Answer from the drawing. Dimensions are ordinates in mm from the lowest x, y and z of the part. Coordinates: 2 decimals unless noted, no trailing zeros. Write each loop counter-clockwise with the first axis right and the second up, starting at its lowest first coordinate (ties: lowest second). Pieces come first, ordered by that corner, then holes.
(1) Section A-A on y = 97.5 is taken. Write down the section's boundary in (x, z), then the cut area to 3 significant figures.
(2) Given pin 1 (3 mm diameter, centred on y = 81.5, z = 403, fed in from +X); pin 2 (4 mm diameter, centred on x = 120.5, z = 214, fed in from +Y), each flat-ended and moving along its own axis, determine where each tip first touches the part or whether it passes through.
(3) Section C-C on z = 207 is taken. Write down the section's boundary in (x, y), then the cut area to 3 significant figures.
(4) Find the intervals of material crossed by probe 1 along Y at (x, z) = (65, 88); probe 2 along Z at (x, y) = (142, 45.5); probe 3 along Z at (x, y) = (118, 10), in increasing order.
(5) Section B-B on x = 33 is taken. Write down the section's boundary in (y, z), then the cut area to 3 significant figures.
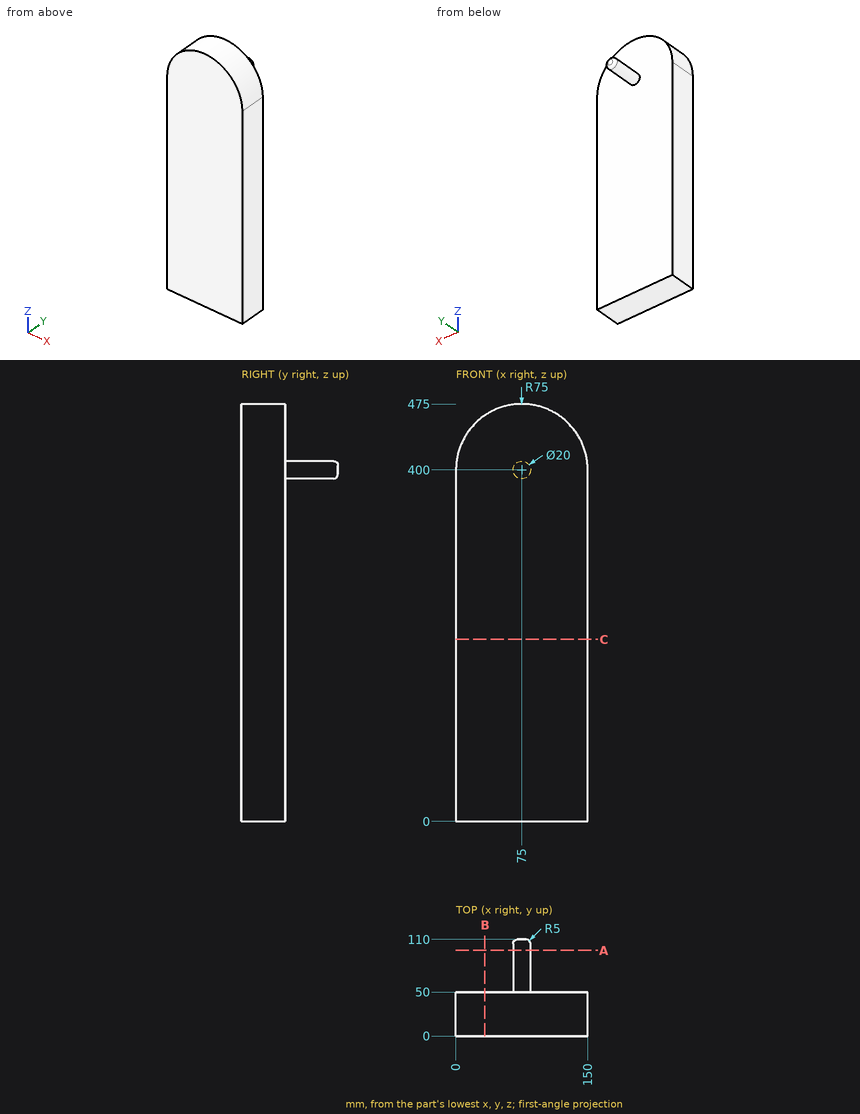
Response:
1. outline: circle Ø20 at (75, 400)
1. area: 314 mm2
2. pin 1: stops at x = 84.89
2. pin 2: stops at y = 50
3. outline: (0, 0) - (150, 0) - (150, 50) - (0, 50) - close
3. area: 7,500 mm2
4. probe 1: y = 0 to 50
4. probe 2: z = 0 to 433.7
4. probe 3: z = 0 to 461.45
5. outline: (0, 0) - (50, 0) - (50, 462.14) - (0, 462.14) - close
5. area: 23,100 mm2
